Input: part model. Units: mm. Frame: model coordinates. Face numbers are marked on the shaded views. A direction names the side the tool comes from. Round coordinates to 2 decimals unless told otherwise and drop trailing zeros. Write each loop counter-clockwise with the first axis right and the second up, starting at its lowest first coordinate (ties: lowest second). Pieces come first, ordered by that corner, then holes. Notation, with made-up numbers: (21.25, 48) - (37.25, 48) arc R11 cw to (37.25, 60) - close; hole circle Ø10 at (25.5, 73.5). An arc over 180 degrees is marked (long way). Use one line per item in the form item = value.
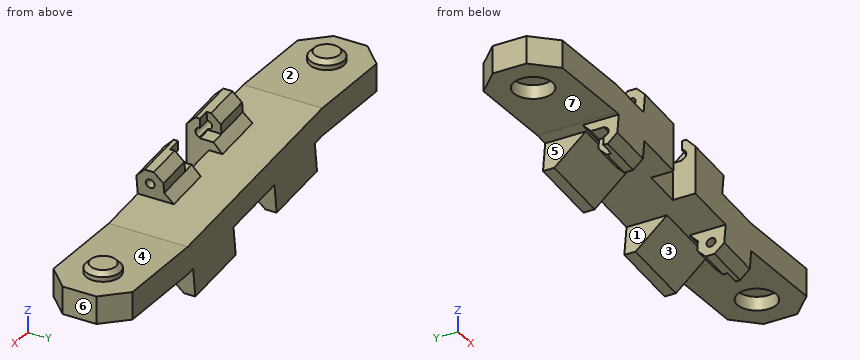
```python
from build123d import *

# Parameters (mm, degrees)
BOSS_EXTRUDE4_DEPTH      = 2.4
BOSS_EXTRUDE4_2_DEPTH    = 2.4
BOSS_EXTRUDE4_3_DEPTH    = 2.4
BOSS_EXTRUDE4_4_DEPTH    = 2.4
BOSS_EXTRUDE5_DEPTH      = 7
SKETCH2_R                = 1.499999999999997
BOSS_EXTRUDE8_DEPTH      = 0.8
SKETCH3_R                = 1.5000000000000007
BOSS_EXTRUDE9_DEPTH      = 0.8
SKETCH4_R                = 1.6999999999999995
CUT_EXTRUDE3_DEPTH       = 1.2
SKETCH5_R                = 1.6999999999999995
CUT_EXTRUDE4_DEPTH       = 1.2
CHAMFER4_SIZE            = 2
CUT_EXTRUDE7_REACH       = 33.32
SKETCH8_R                = 0.3999999999999905
SKETCH8_R_2              = 0.4000000000000032
CUT_EXTRUDE10_DEPTH      = 2
CHAMFER6_SIZE            = 0.8
CUT_EXTRUDE11_DEPTH      = 10
CUT_EXTRUDE11_DEPTH_BACK = 1.2
BOSS_EXTRUDE10_DEPTH     = 3.6
CHAMFER8_SIZE            = 2.6
CHAMFER9_SIZE            = 0.4


with BuildPart() as part:
    # Sketch1 → Boss-Extrude4 (new body)
    with BuildSketch(Plane(origin=(0, 0, 0), x_dir=(1, 0, 0), z_dir=(0, 1, 0))):
        Polygon((-6.033824051637797, -1.9503087992717978), (-5.721324051637796, -4.430700653394863), (-1.5999999999999996, -3.911462628969018), (-1.5999999999999994, -1.3916994755741596), align=None)
    extrude(amount=BOSS_EXTRUDE4_DEPTH)



with BuildPart() as body_2:
    # Sketch1 → Boss-Extrude4 2 (new body)
    with BuildSketch(Plane(origin=(0, 0, 0), x_dir=(1, 0, 0), z_dir=(0, 1, 0))):
        Polygon((-10.000000000000064, 2.4499999999999993), (-9.689951018234682, -0.01093750000000027), (-5.919755399967642, 0.4640624999999997), (-6.229804381733024, 2.9250000000000003), align=None)
    extrude(amount=BOSS_EXTRUDE4_2_DEPTH)


with BuildPart() as body_3:
    # Sketch1 → Boss-Extrude4 3 (new body)
    with BuildSketch(Plane(origin=(0, 0, 0), x_dir=(1, 0, 0), z_dir=(0, 1, 0))):
        Polygon((5.564458884622125, -0.4890625000000022), (1.6000000000000032, -0.9885373710309839), (1.6000000000000008, -3.508300524425846), (5.876958884622125, -2.969454354123069), align=None)
    extrude(amount=BOSS_EXTRUDE4_3_DEPTH)


with BuildPart() as body_4:
    # Sketch1 → Boss-Extrude4 4 (new body)
    with BuildSketch(Plane(origin=(0, 0, 0), x_dir=(1, 0, 0), z_dir=(0, 1, 0))):
        Polygon((5.7628902329519684, 4.435937500000006), (6.072939214717352, 1.9750000000000023), (9.843134832984354, 2.4499999999999993), (9.533085851218969, 4.910937500000012), align=None)
    extrude(amount=BOSS_EXTRUDE4_4_DEPTH)


with BuildPart() as part_1:
    add(part.part)

    add(body_2.part)  # Boss-Extrude5 merges body 2

    add(body_3.part)  # Boss-Extrude5 merges body 3

    add(body_4.part)  # Boss-Extrude5 merges body 4
    # Sketch1<8> → Boss-Extrude5 (add)
    with BuildSketch(Plane(origin=(0, 0, 0), x_dir=(1, 0, 0), z_dir=(0, 1, 0))):
        Polygon((-20, -0.05000000000000027), (-20, -2.45), (-12, -2.4499999999999997), (-10.000000000000064, -2.4499999999999997), (-6.033824051637797, -1.950308799271796), (-1.9124999999999996, -1.431070774845953), (-1.6000000000000032, -1.391699475574159), (-1.5999999999999999, 1.0083005244258434), (-5.919755399967642, 0.4640624999999997), (-9.689951018234682, -0.01093750000000025), (-10.000000000000064, -0.05000000000000029), (-12, -0.05000000000000027), align=None)
        Polygon((1.6000000000000003, 1.4114626289690202), (1.6000000000000005, -0.988537371030981), (5.564458884622125, -0.4890625000000022), (9.687500000000064, 0.03039185412306233), (9.843134832984425, 0.05000000000000027), (12, 0.05000000000000013), (20, 0.05000000000000013), (20, 2.4499999999999997), (12, 2.4499999999999993), (9.843134832984353, 2.4499999999999993), (6.072939214717351, 1.975000000000004), (1.9100489817653816, 1.4505251289690204), align=None)
        Polygon((-1.5999999999999999, 1.0083005244258434), (-1.5999999999999994, -1.3916994755741596), (1.6000000000000032, -0.9885373710309839), (1.6000000000000003, 1.4114626289690202), align=None)
    extrude(amount=BOSS_EXTRUDE5_DEPTH)

    # Sketch2 → Boss-Extrude8 (add)
    with BuildSketch(Plane.XY.offset(2.4499999999999993)):
        with Locations(Location((-16.5, 3.4999999999999996, 0), (0, 0, 180))):
            Circle(SKETCH2_R)
    extrude(amount=BOSS_EXTRUDE8_DEPTH)

    # Sketch3 → Boss-Extrude9 (add)
    with BuildSketch(Plane.XY.offset(-0.05000000000000013)):
        with Locations(Location((16.5, 3.4999999999999996, 0), (0, 0, 180))):
            Circle(SKETCH3_R)
    extrude(amount=BOSS_EXTRUDE9_DEPTH)

    # Sketch4 → Cut-Extrude3 (cut)
    with BuildSketch(Plane(origin=(0, 0, 0.05000000000000041), x_dir=(-1, 0, -5e-17), z_dir=(5e-17, 0, -1))):
        with Locations((16.5, 3.4999999999999996)):
            Circle(SKETCH4_R)
    extrude(amount=-CUT_EXTRUDE3_DEPTH, mode=Mode.SUBTRACT)

    # Sketch5 → Cut-Extrude4 (cut)
    with BuildSketch(Plane(origin=(-1e-16, 0, -2.449999999999999), x_dir=(-1, 0, 5e-17), z_dir=(-5e-17, 0, -1))):
        with Locations((-16.5, 3.4999999999999996)):
            Circle(SKETCH5_R)
    extrude(amount=-CUT_EXTRUDE4_DEPTH, mode=Mode.SUBTRACT)

    # Chamfer4
    chamfer4_edges = [part_1.edges().sort_by_distance(p)[0] for p in [
        (20, 7, -1.25),
        (-20, 7, 1.2500000000000002),
        (-20, 0, 1.2500000000000002),
        (20, 0, -1.25),
    ]]
    chamfer(chamfer4_edges, length=CHAMFER4_SIZE)

    # Cut-Extrude7: up to this face of the body (flat: up to its plane)
    cut_extrude7_end = Plane(part_1.part.faces().sort_by_distance((-9.844975509, 1.2, -1.21953125))[0])
    # Sketch8 → Cut-Extrude7 (cut, up to the picked face)
    with BuildSketch(Plane(origin=(9.99318385334905, 0, -1.2590228229384695), x_dir=(-0.12500000000000053, 0, -0.9921567416492215), z_dir=(0.9921567416492215, 0, -0.12500000000000053)), mode=Mode.PRIVATE) as cut_extrude7_sk1:
        with Locations((2.4807840170405906, 1.2000000000000017)):
            Circle(SKETCH8_R)
    cut_extrude7_tool1 = split(extrude(cut_extrude7_sk1.sketch, amount=-CUT_EXTRUDE7_REACH, mode=Mode.PRIVATE), bisect_by=cut_extrude7_end, keep=Keep.BOTH, mode=Mode.PRIVATE)
    # Sketch8 → Cut-Extrude7 (cut, up to the picked face)
    with BuildSketch(Plane(origin=(9.99318385334905, 0, -1.2590228229384695), x_dir=(-0.12500000000000053, 0, -0.9921567416492215), z_dir=(0.9921567416492215, 0, -0.12500000000000053)), mode=Mode.PRIVATE) as cut_extrude7_sk2:
        with Locations((-2.4807840170405973, 1.200000000000001)):
            Circle(SKETCH8_R_2)
    cut_extrude7_tool2 = split(extrude(cut_extrude7_sk2.sketch, amount=-CUT_EXTRUDE7_REACH, mode=Mode.PRIVATE), bisect_by=cut_extrude7_end, keep=Keep.BOTH, mode=Mode.PRIVATE)
    add(cut_extrude7_tool1.solids().sort_by(Axis((9.683086, 1.2, -3.720349), (-0.9921567416492215, 0, 0.12500000000000053)))[0], mode=Mode.SUBTRACT)
    add(cut_extrude7_tool2.solids().sort_by(Axis((10.303282, 1.2, 1.202304), (-0.9921567416492215, 0, 0.12500000000000053)))[0], mode=Mode.SUBTRACT)

    # Sketch1<10> → Cut-Extrude10 (cut)
    with BuildSketch(Plane(origin=(0, 0, 0), x_dir=(1, 0, 0), z_dir=(0, 1, 0))):
        Polygon((-1.5999999999999999, 1.0083005244258434), (-1.5999999999999994, -1.3916994755741596), (1.6000000000000032, -0.9885373710309839), (1.6000000000000003, 1.4114626289690202), align=None)
        Polygon((-1.6, 3.5083005244258283), (-1.5999999999999999, 1.0083005244258434), (1.5999999999999979, 1.4114626289690202), (1.6, 3.9114626289690166), align=None)
        Polygon((1.6000000000000032, -0.9885373710309839), (-1.6000000000000032, -1.391699475574159), (-1.5999999999999992, -3.91146262896902), (1.6000000000000014, -3.5083005244258425), align=None)
    extrude(amount=CUT_EXTRUDE10_DEPTH, mode=Mode.SUBTRACT)

    # Chamfer6
    chamfer6_edges = [part_1.edges().sort_by_distance(p)[0] for p in [
        (-3.816912025818899, 2.4, 1.6710041374229787),
        (-3.660662025818898, 2.4, 4.17108164118194),
        (3.738479442311063, 0, 3.2388774392744577),
        (3.582229442311064, 2.4, 0.7387999355154931),
        (3.738479442311063, 2.4, 3.2388774392744577),
        (7.647988042085475, 2.4, -4.673437499999995),
        (7.958037023850853, 2.4, -2.2125000000000017),
        (7.647988042085475, 0, -4.673437499999995),
        (-3.660662025818898, 0, 4.17108164118194),
        (-8.114902190866543, 2.4, -2.6874999999999987),
        (-7.804853209101163, 2.4, -0.22656249999999975),
        (-8.114902190866543, 0, -2.6874999999999987),
    ]]
    chamfer(chamfer6_edges, length=CHAMFER6_SIZE)

    # Sketch9 → Cut-Extrude11 (cut, two sides: drawn at the far end of the back side and taken through both)
    with BuildSketch(Plane(origin=(0, 2.4, 0), x_dir=(1, 0, 0), z_dir=(0, 1, 0)).offset(-CUT_EXTRUDE11_DEPTH_BACK)):
        Polygon((-10.000000000000064, 2.4499999999999984), (-9.789951018234682, 0.7827878933193786), (-8.599362928255616, 0.9327878933193787), (-8.809411910021, 2.5999999999999988), align=None)
        Polygon((-1.5999999999999994, -2.198023684660508), (-2.7905880899790625, -2.348023684660507), (-2.578088089979061, -4.0346901454641975), (-1.3874999999999975, -3.884690145464198), align=None)
        Polygon((1.6000000000000008, -3.508300524425844), (1.3874999999999984, -1.8216340636221509), (2.5780880899790635, -1.671634063622151), (2.790588089979066, -3.3583005244258444), align=None)
        Polygon((9.533085851218972, 4.910937499999992), (8.342497761239906, 4.760937499999993), (8.552546743005287, 3.0937253933193816), (9.743134832984353, 3.2437253933193815), align=None)
    extrude(amount=CUT_EXTRUDE11_DEPTH + CUT_EXTRUDE11_DEPTH_BACK, mode=Mode.SUBTRACT)

    # Sketch10 → Boss-Extrude10 (add)
    with BuildSketch(Plane(origin=(0, 6.999999999999999, 0), x_dir=(1, 0, 0), z_dir=(0, 1, 0))):
        Polygon((8.724409439665015, 4.929607528287985), (2.7714689897696854, 4.179607528287982), (3.0964689897696878, 1.600000000000004), (9.04940943966502, 2.3500000000000094), align=None)
        Polygon((-9.221225624915308, 2.6686700282879747), (-8.896225624915308, 0.08906249999999957), (-2.943285175019977, 0.8390625000000002), (-3.2682851750199777, 3.418670028287977), align=None)
    extrude(amount=-BOSS_EXTRUDE10_DEPTH)

    # Chamfer8
    chamfer8_edges = [part_1.edges().sort_by_distance(p)[0] for p in [
        (-6.244755399967643, 3.399999999999999, -3.0436700282879756),
        (5.74793921471735, 3.399999999999999, -4.554607528287983),
    ]]
    chamfer(chamfer8_edges, length=CHAMFER8_SIZE - 0.0001)  # a hair under: the kernel refuses the full size

    # Chamfer9
    chamfer9_edges = [part_1.edges().sort_by_distance(p)[0] for p in [
        (-15.000000000000004, 3.499999999999999, 3.249999999999999),
        (18, 3.499999999999999, 0.7499999999999999),
    ]]
    chamfer(chamfer9_edges, length=CHAMFER9_SIZE)


solid = part_1.part
```
(1) First-contact query: pin 1 Ø3.5 at (x, y) = (-16.5, 2) entering from +Z; pin 2 Ø1.5 at (x, y) = (-12, 6) entering from -Z; pin 3 Ø1 at (x, y) = (15.5, 3.5) entering from -Z; pin 4 Ø2.5 at (y, z) = (1, 0.5) entering from -X. Flat tips, straight axial feed; report the tip coordinate or a pass-through.
Derived:
pin_1 = 3.25
pin_2 = 0.05
pin_3 = -1.25
pin_4 = -20
(2) Material intervals for L1, parallel to Y at x = 16.5, z = -2; L2, parallel to Z at x = -16.5, y = 3.5; L3, parallel to Y at x = -2.5, z = 2.75, sorted ascending.
Derived:
L1 = 0 to 1.8, 5.2 to 7
L2 = 1.25 to 3.25
L3 = 0 to 0.81
(3) Cut plane A-A on x = -16.5. Output: boundary loops of the cut face in (y, z).
Derived:
outline = (0, 0.05) - (1.8, 0.05) - (1.8, 1.25) - (5.2, 1.25) - (5.2, 0.05) - (7, 0.05) - (7, 2.45) - (5, 2.45) - (5, 2.85) - (4.6, 3.25) - (2.4, 3.25) - (2, 2.85) - (2, 2.45) - (0, 2.45) - close
(4) Draft query along Z for the marked faces 4, 5, 6 and 7. Return one class per face: released by +Z, released by -Z, zero draft, split by the parting line, or undercut.
Derived:
face_4 = released by +Z
face_5 = undercut
face_6 = zero draft
face_7 = released by -Z
(5) Access query for the marked faces 1, 2 and 3. Directions: +Z, -Z, +X, -X, +Y, -Y. A direction counts if a zero-diameter tool reaches every point of the face in a straight line with its end or side. Return the directions, or none.
Derived:
face_1 = +Y, -Y
face_2 = +Z
face_3 = -Z, -X
